Autodesk Inventor part; units mm, degrees
ref_plane "YZ Plane" through (0, 0, 0) normal (1, 0, 0) x (0, 1, 0)
ref_plane "XZ Plane" through (0, 0, 0) normal (0, 1, 0) x (-1, 0, 0)
ref_plane "XY Plane" through (0, 0, 0) normal (0, 0, 1) x (1, 0, 0)
sketch "Sketch1" plane through (0, 0, 0) normal (0, 0, 1) x (1, 0, 0)
  line L0 (10, 3) -> (35, 3)
  line L1 (10, 0) -> (10, 3)
  line L2 (35, 0) -> (10, 0)
  line L3 (35, 0) -> (35, 3)
  line L4 (0, 3) -> (10, 3)
  line L5 (-3, 10) -> (-3, 15)
  line L6 (0, 15) -> (-3, 15)
  line L7 (0, 15) -> (0, 25)
  line L8 (35, 3) -> (45, 3)
  line L9 (45, 10) -> (45, 0)
  line L10 (48, 10) -> (45, 10)
  line L11 (48, 15) -> (48, 10)
  line L12 (45, 15) -> (48, 15)
  line L13 (45, 25) -> (45, 15)
  line L14 (0, 25) -> (5, 25)
  line L15 (5, 25) -> (5, 22)
  line L16 (5, 22) -> (0, 22)
  line L17 (0, 22) -> (0, 25)
  line L18 (45, 25) -> (40, 25)
  line L19 (40, 25) -> (40, 22)
  line L20 (40, 22) -> (45, 22)
  line L21 (45, 22) -> (45, 25)
  line L22 (5, 22) -> (40, 22)
  circle A0 centre (6.5, 7) radius 4
  circle A1 centre (6.5, 7) radius 2.5
  line L23 (0, 10) -> (-3, 10)
  line L24 (0, 0) -> (0, 10)
  dimension "d0" = 5
  dimension "d1" = 3
  dimension "d2" = 5
  dimension "d3" = 3
  dimension "d4" = 5
extrude "Extrusion1" add sketch "Sketch1" along normal blind 3 contours A0 | L4 L24 L23 L5 L6 L7 L16 L22 L20 L13 L12 L11 L10 L9 L8 L0 | L0 L3 L2 L1 | L20 L19 L18 L13 | L7 L14 L15 L16
properties part number "SideTopNM" material "Acrylic, Clear"
CAD build for the part. Positions are in the model's coordinates, mm. A direction names the side the tool comes from. Round coordinates to 2 decimals unless told otherwise and drop trailing zeros. Order: outer loops, then holes, each group sorted by start corner. A loop starts at its lowest first (then second) coordinate and runs counter-clockwise, first axis right, second up. Notation, with made-up numbers: (-35.5, 58) - (-3.5, 58) arc R30 cw to (-3.5, 87) - close; hole circle Ø8 at (85.5, 79.25). An arc over 180 degrees is marked (long way). Use CSV: the item, a comma, the result in double quotes. Start each with the question number.
1) Saw through at D-D (x = 23). List the corners of the cut face in (y, z), and give its area (3 significant figures).
2) Saw through at A-A (x = 6.5). List the corners of the cut face in (y, z), and give its area (3 significant figures).
3) Two-plate mould, pull along Y, no slides. Class faces 1 (the cylindrical face through (8.81, 7.96, 1.48)), 2 (the flat face through (47, 10, 1)), 3 (the flat face through (45, 20, 1)), 4 (the flat face through (22, 22, 1)): pulls with the +Y half, pulls with the -Y half, needs draft (parallel to the pull), parting line crosses it, or undercut.
4) Saw through at B-B (z = 2.2). List the corners of the cut face in (x, y), and give its area (3 significant figures).
5) Pin check, flat tips, straight feed: pin 1 Ø0.9 at (x, z) = (-1.5, 1.5) entering from +Y; pin 2 Ø1.5 at (y, z) = (1.5, 2) entering from +X; pin 3 Ø0.9 at (y, z) = (23, 1) entering from +X; pin 4 Ø4 at (x, y) = (6.5, 7) entering from +Z. Stop position of each tip, or through.
6) Tool access for faces 5 (the flat face through (46, 15, 1)), 6 (the flat face through (35, 1, 1)), 7 (the flat face through (0, 6, 1)), 8 (the flat face through (0, 20, 1)): list every direction of +Z, -Z, +X, -X, +Y, -Y with a clear straight run to the whole face (end or side of a thin tool).
7) Wall check: L1, parallel to Y at x = 6.5, z = 1.8; L2, parallel to Y at x = 14, z = 2.15; L3, parallel to Y at x = -1, z = 0.25. Give the ranges that are in metal, low to high. Write a range as [from, to].
8) Saw through at C-C (y = 7). List the corners of the cut face in (x, z), and give its area (3 significant figures).
Values follow:
1,outline,"(0, 0) - (22, 0) - (22, 3) - (0, 3) - close"
1,area,"66.0 mm2"
2,outline,"(3, 0) - (4.5, 0) - (4.5, 3) - (3, 3) - close; (9.5, 0) - (22, 0) - (22, 3) - (9.5, 3) - close"
2,area,"42.0 mm2"
3,face 1,"undercut"
3,face 2,"pulls with the -Y half"
3,face 3,"needs draft"
3,face 4,"pulls with the +Y half"
4,outline,"(-3, 10) - (0, 10) - (0, 3) - (10, 3) - (10, 0) - (35, 0) - (35, 3) - (45, 3) - (45, 10) - (48, 10) - (48, 15) - (45, 15) - (45, 25) - (40, 25) - (40, 22) - (5, 22) - (5, 25) - (0, 25) - (0, 15) - (-3, 15) - close; hole circle Ø5 at (6.5, 7)"
4,area,"970 mm2"
5,pin 1,"stops at y = 15"
5,pin 2,"stops at x = 35"
5,pin 3,"stops at x = 45"
5,pin 4,"passes through"
6,face 5,"+Z, -Z, +X, +Y"
6,face 6,"+Z, -Z, +X, -Y"
6,face 7,"+Z, -Z, -X, -Y"
6,face 8,"+Z, -Z, -X, +Y"
7,L1,"y = [3, 4.5], [9.5, 22]"
7,L2,"y = [0, 22]"
7,L3,"y = [10, 15]"
8,outline,"(0, 0) - (4, 0) - (4, 3) - (0, 3) - close; (9, 0) - (45, 0) - (45, 3) - (9, 3) - close"
8,area,"120 mm2"
